Could you check a few things on this drawing? It's one solid part, dimensions in mm from its lowest x, y, z. Round coordinates to 2 decimals unless told otherwise and drop trailing zeros. Order: outer loops, then holes, each group sorted by start corner. A loop starts at its lowest first (then second) coordinate and runs counter-clockwise, first axis right, second up. Notation, with made-up numbers: (-34.75, 66) -> (19.25, 66) arc R19 ccw to (19.25, 83) -> close; hole circle Ø4 at (-14.75, -6.75). An arc over 180 degrees is marked (long way). Use a Markdown table: item, result. Add a question column.
(1) I want a section at B-B, the plane z = 96.5. Please give me the cut outline in (x, y), then the cut area to 3 significant figures.
(2) I want a section at A-A, the plane x = 1.7. Please give me the cut outline in (y, z) (3 decimals).
(3) If I drill on probe 1 along Z at (x, y) = (2.9, 1.5); probe 2 along Y at (x, z) = (4.4, 16.5); probe 3 along Y at (x, z) = (3.4, 73), over which ranges is the centre line in solid material (lowest first)?
(4) I want a section at C-C, the plane y = 22.25. Please give me the cut outline in (x, z) (3 decimals), then the cut area to 3 significant figures.
(5) I'm going to push flat-ended pins straight in: P1, Ø1.4, axis at x = 3, y = 2, coming from the -Z side; P2, Ø2.5, axis at x = 3.5, y = 3.5, coming from the +Z side; P3, Ø1, axis at x = 4, z = 28, coming from the +Y side. Where does each tip first touch, or does it pass through?
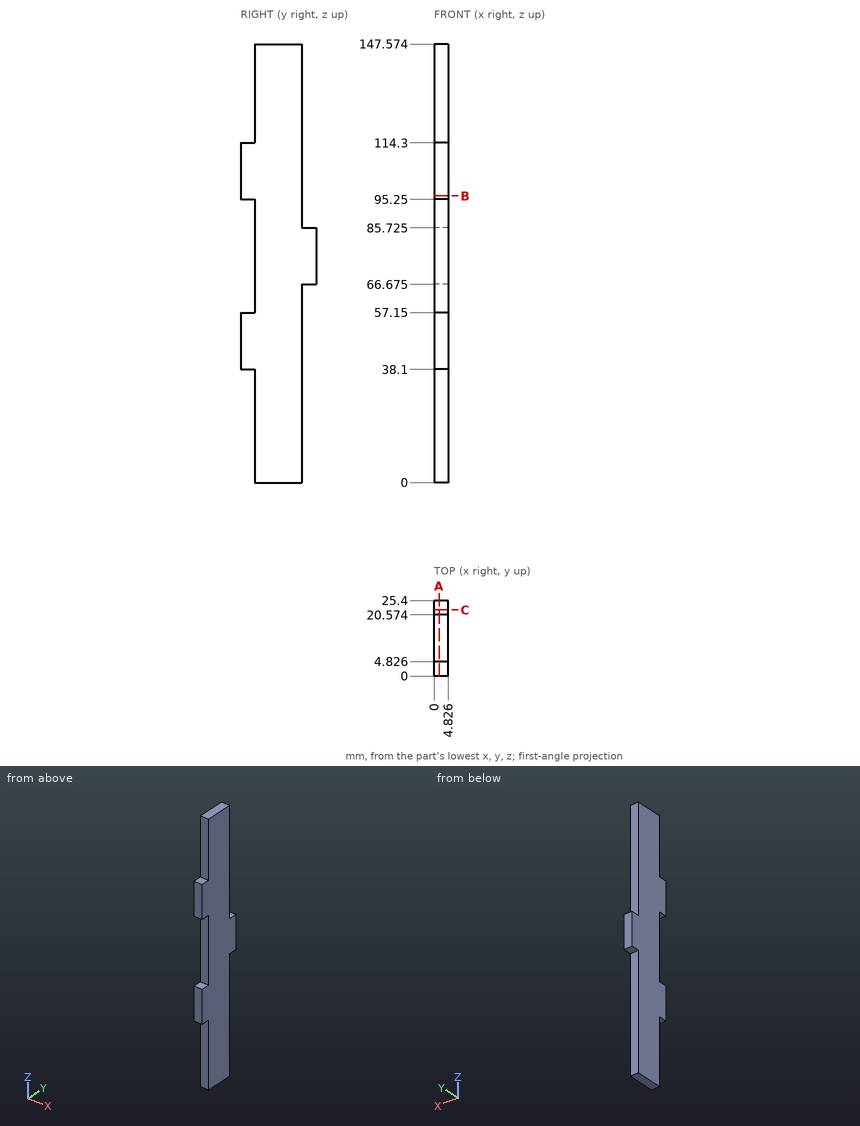
Taken from the geometry:
| question | item | result |
|---|---|---|
| 1 | outline | (0, 0) -> (4.83, 0) -> (4.83, 20.57) -> (0, 20.57) -> close |
| 1 | area | 99.3 mm2 |
| 2 | outline | (0, 38.1) -> (4.826, 38.1) -> (4.826, 0) -> (20.574, 0) -> (20.574, 66.675) -> (25.4, 66.675) -> (25.4, 85.725) -> (20.574, 85.725) -> (20.574, 147.574) -> (4.826, 147.574) -> (4.826, 114.3) -> (0, 114.3) -> (0, 95.25) -> (4.826, 95.25) -> (4.826, 57.15) -> (0, 57.15) -> close |
| 3 | probe 1 | z = 38.1 to 57.15, 95.25 to 114.3 |
| 3 | probe 2 | y = 4.83 to 20.57 |
| 3 | probe 3 | y = 4.83 to 25.4 |
| 4 | outline | (0, 66.675) -> (4.826, 66.675) -> (4.826, 85.725) -> (0, 85.725) -> close |
| 4 | area | 91.9 mm2 |
| 5 | P1 | stops at z = 38.1 |
| 5 | P2 | stops at z = 114.3 |
| 5 | P3 | stops at y = 20.57 |
